Print and shaded views of the part. All mm, measured from the part's lowest x, y and z. A direction names the side the tool comes from. Give positions to 0.01 mm unless a question says otherwise; leave off trailing zeros. Order: outer loops, then holes, each group sorted by start corner. A loop starts at its lowest first (then second) coordinate and runs counter-clockwise, first axis right, second up. Notation, with made-up numbers: (-32.75, -1) - (-20.75, -1) arc R27 cw to (-20.75, 36) - close; hole circle Ø2 at (-26, -4). An arc over 180 degrees is marked (long way). Answer in a Markdown table with one row per item.
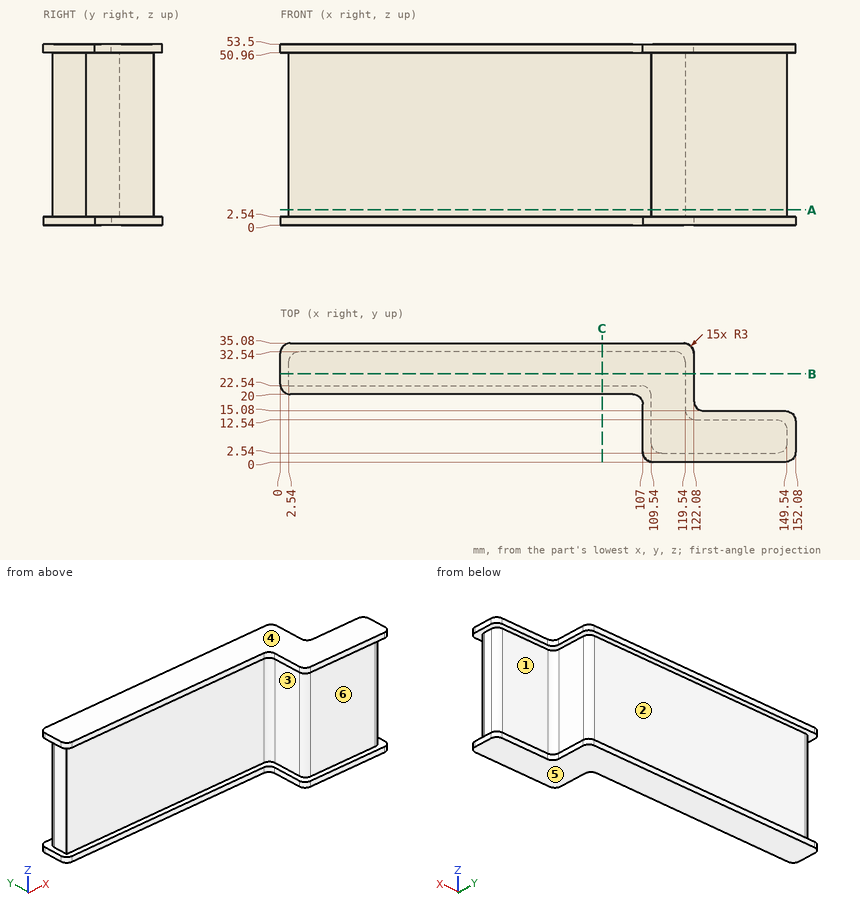
1. Cut at C-C on x = 95. Write the cut outline in (y, z), and give its area (3 significant figures).
Check result:
| item | result |
|---|---|
| outline | (20, 0) - (35.08, 0) - (35.08, 2.54) - (32.54, 2.54) - (32.54, 50.96) - (35.08, 50.96) - (35.08, 53.5) - (20, 53.5) - (20, 50.96) - (22.54, 50.96) - (22.54, 2.54) - (20, 2.54) - close |
| area | 561 mm² |
2. Cut at B-B on y = 26. Write the cut outline in (x, z).
Check result:
| item | result |
|---|---|
| outline | (0, 0) - (122.08, 0) - (122.08, 2.54) - (119.54, 2.54) - (119.54, 50.96) - (122.08, 50.96) - (122.08, 53.5) - (0, 53.5) - (0, 50.96) - (2.54, 50.96) - (2.54, 2.54) - (0, 2.54) - close |
3. Probe line 1 (Y direction, x = 66, z = 20.5); line 2 (X direction, y = 6.5, z = 4); line 3 (X direction, y = 6, z = 2). List the from-to ranges inside material, lowest first.
Check result:
| item | result |
|---|---|
| line 1 | y = 22.54 to 32.54 |
| line 2 | x = 109.54 to 149.54 |
| line 3 | x = 107 to 152.08 |
4. Cut at A-A on z = 4.5. Write the cut outline in (x, y), and give its area (3 significant figures).
Check result:
| item | result |
|---|---|
| outline | (2.54, 22.54) - (106.54, 22.54) arc R3 cw to (109.54, 19.54) - (109.54, 5.54) arc R3 ccw to (112.54, 2.54) - (146.54, 2.54) arc R3 ccw to (149.54, 5.54) - (149.54, 9.54) arc R3 ccw to (146.54, 12.54) - (122.54, 12.54) arc R3 cw to (119.54, 15.54) - (119.54, 29.54) arc R3 ccw to (116.54, 32.54) - (5.54, 32.54) arc R3 ccw to (2.54, 29.54) - close |
| area | 1,660 mm² |
5. Which spindle directions (+Z, -Z, +X, -X, +Y, -Y) get a long thin tool onto all of the face, cutting with end or side? Do the marked faces 1, 2 and 3. Say none if no direction does.
Check result:
| item | result |
|---|---|
| face 1 | +X, +Y |
| face 2 | +X, -X, +Y |
| face 3 | -X, -Y |
6. Two-plate mould, pull along Z, no slides. Class the marked faces 4, 5 and 6: +Z half, -Z half, draft (parallel to the pull), parting line (faces both ways), or undercut.
Check result:
| item | result |
|---|---|
| face 4 | +Z half |
| face 5 | -Z half |
| face 6 | undercut |
7. Drop flat-ended pins along their axis: P1, Ø0.8, axis at x = 142, z = 1.5, coming from the +Y side; P2, Ø10, axis at y = 13, z = 15, coming from the -X side; P3, Ø3, axis at y = 27.5, z = 0.5, coming from the +X side. Give the stop position or say it passes through.
Check result:
| item | result |
|---|---|
| P1 | stops at y = 15.08 |
| P2 | stops at x = 109.54 |
| P3 | stops at x = 122.08 |
